```python
from build123d import *

# Parameters (mm, degrees)
F0_W     = 50.8
F0_H     = 12.7
F1_DEPTH = 3.175
F2_R     = 3.175
F3_DEPTH = 6.35
F5_DEPTH = 6.35
F6_R     = 3.175
F7_R     = 6.34999


# Not quite as in the source:
# - a fillet or chamfer is up to 0.001 mm smaller than in the source, because OpenCascade refuses the exact size


with BuildPart() as f1:
    # F0 (on Front) → F1 (new body)
    with BuildSketch(Plane.XZ):
        with Locations((25.4, 6.35)):
            Rectangle(F0_W, F0_H)
    extrude(amount=F1_DEPTH)

    # F2 (on face) → F3 (join)
    with BuildSketch(Plane.XZ.offset(3.175)):
        with Locations((38.1, 6.35)):
            Circle(F2_R)
    extrude(amount=F3_DEPTH)

    # F4 (on face) → F5 (join)
    with BuildSketch(Plane(origin=(0, 0, 0), x_dir=(-1, 0, 0), z_dir=(0, 1, 0))):
        Polygon((0, 0), (0, 12.7), (-25.4, 12.7), (-25.4, 10.795), (-1.905, 10.795), (-1.905, 1.905), (-25.4, 1.905), (-25.4, 0), align=None)
    extrude(amount=F5_DEPTH)

    # F6
    f6_edges = [f1.edges().sort_by_distance(p)[0] for p in [
        (1.905, 3.175, 10.795),
        (1.905, 3.175, 1.905),
    ]]
    fillet(f6_edges, radius=F6_R)

    # F7 (radius 6.35 in the source; OpenCascade refuses exactly that, so slightly less here)
    f7_edges = [f1.edges().sort_by_distance(p)[0] for p in [
        (50.8, -1.5875, 12.7),
        (50.8, -1.5875, 0),
    ]]
    fillet(f7_edges, radius=F7_R)


solid = f1.part
```
The model under review builds one solid part; all positions refer to its coordinate system, in mm. A direction names the side the tool comes from. Give positions to 0.01 mm unless a question says otherwise; leave off trailing zeros. Loops run counter-clockwise (first coordinate to the right, second up) from the corner with the lowest first, then second, coordinate; pieces in that order, holes last. Notation, with made-up numbers: (65.25, 57.5) - (91.25, 57.5) arc R18 cw to (91.25, 61.5) - close; hole circle Ø6 at (-39.5, 36). An arc over 180 degrees is marked (long way). Answer as a JSON object with one key per item and string values.
Q1. Add section D-D on x = 19. State the section outline as (y, z) points (3 decimals), plus the area to 3 significant figures.
Worked out:
{"outline": "(-3.175, 0) - (6.35, 0) - (6.35, 1.905) - (0, 1.905) - (0, 10.795) - (6.35, 10.795) - (6.35, 12.7) - (-3.175, 12.7) - close", "area": "64.5 mm^2"}
Q2. Insertion check: pin 1 (6 mm diameter, centred on x = 28.5, z = 2.5, fed in from -Y) (3 decimals); pin 2 (1.3 mm diameter, centred on y = 4, z = 6, fed in from +X) (3 decimals); pin 3 (3 mm diameter, centred on y = -6, z = 7, fed in from -X) (3 decimals). Each pin has a flat end and moves straight along its axis. Give the tip position at first contact, or say it passes through.
Worked out:
{"pin 1": "stops at y = -3.175", "pin 2": "stops at x = 1.905", "pin 3": "stops at x = 34.925"}
Q3. To check wall thickness, follow line 1 along X through (y, z) = (4.5, 11); line 2 along Y through (x, z) = (39.5, 12) (3 decimals); line 3 along Y through (x, z) = (2, 11.25) (3 decimals). State the ranges of each line that lie inside material, in increasing order.
Worked out:
{"line 1": "x = 0 to 25.4", "line 2": "y = -3.175 to 0", "line 3": "y = -3.175 to 6.35"}
Q4. Mouldability with a two-part tool opening along Z and no side actions: class faces 5 (the flat face through (38, -9.525, 6)), 6 (the flat face through (17, 0, 12.7)), 7 (the flat face through (15, 3, 1.905)) as +Z half, -Z half, draft (parallel to the pull), parting line (faces both ways), or undercut.
Worked out:
{"face 5": "draft", "face 6": "+Z half", "face 7": "undercut"}
Q5. Add section A-A on x = 38.1. State the section outline as (y, z) points (3 decimals), plus the area to 3 significant figures.
Worked out:
{"outline": "(-9.525, 3.175) - (-3.175, 3.175) - (-3.175, 0) - (0, 0) - (0, 12.7) - (-3.175, 12.7) - (-3.175, 9.525) - (-9.525, 9.525) - close", "area": "80.6 mm^2"}
Q6. For faces 1 (the cylindrical face through (48.89, -1.61, 1.81)), 2 (the flat face through (25.4, 3, 1)), 3 (the cylindrical face through (35.76, -6.306, 8.496)), 4 (the cylindrical face through (2.86, 3.22, 9.89)), list the 3-axis set-ups (+Z, -Z, +X, -X, +Y, -Y) from which the entire face can be reached by the end or side of a thin tool; tool diameter is ignored.
Worked out:
{"face 1": "-Z, +X, +Y, -Y", "face 2": "+Z, -Z, +X, +Y", "face 3": "-Y", "face 4": "+X, +Y"}
Q7. Add section C-C on z = 3.75. State the section outline as (x, y) points (3 decimals).
Worked out:
{"outline": "(0, -3.175) - (36.278, -3.175) - (36.278, -9.525) - (39.922, -9.525) - (39.922, -3.175) - (50.243, -3.175) - (50.243, 0) - (2.197, 0) - (2.197, 6.35) - (0, 6.35) - close"}
